from build123d import *

# Parameters (mm, degrees)
F1_DEPTH       = 600
F2_R           = 5
F3_R           = 5
F4_T1_DEPTH    = 611.3695297687
F5_SIZE        = 1
F7_D           = 2.5
F7_CBORE_D     = 6.5
F7_CBORE_DEPTH = 3


# Not quite as in the source:
# - a fillet or chamfer that OpenCascade refuses, or shapes differently, is made with other operations: its cross-section is extruded or revolved along the edge and cut away or added


with BuildPart() as f1:
    # F0 (on Front) → F1 (new body)
    with BuildSketch(Plane.XZ):
        Polygon((-100, 12.6136353192), (0, 12.6136353192), (0, 17.5048394176), (0, 17.6136353192), (-100, 17.6136353192), (-125.63551, 43.2491453192), (-130.63551, 48.2491453192), (-155.818130374, 48.7903356552), (-155.818130374, 43.2491453192), (-130.63551, 43.2491453192), align=None)
    extrude(amount=F1_DEPTH)

    # F2
    f2_edges = [f1.edges().sort_by_distance(p)[0] for p in [
        (-130.63551, -300, 48.249145),
        (-100, -300, 17.613635),
    ]]
    fillet(f2_edges, radius=F2_R)

    # F3
    f3_edges = [f1.edges().sort_by_distance(p)[0] for p in [
        (-130.63551, -300, 43.249145),
        (-100, -300, 12.613635),
        (-155.81813, -300, 43.249145),
    ]]
    fillet(f3_edges, radius=F3_R)

    # F4: fillet of radius 5 on 1 edges, made by hand

    # F4_s2 → F4_t1 (cut)
    with BuildSketch(Plane.XZ.offset(-5.6847648844)):
        with BuildLine():
            ThreePointArc((-155.818130374, 48.2491453192), (-154.7104681905, 48.6293523426), (-153.5447493368, 48.7414792682))
            Line((-153.5447493368, 48.7414792682), (-155.818130374, 48.7903356552))
            Line((-155.818130374, 48.7903356552), (-155.818130374, 48.2491453192))
        make_face()
    extrude(amount=F4_T1_DEPTH, mode=Mode.SUBTRACT)

    # F5
    f5_edges = [f1.edges().sort_by_distance(p)[0] for p in [
        (-48.964466, 0, 17.613635),
        (-48.964466, 0, 12.613635),
        (-115.317755, 0, 27.93139),
        (-130.793161, 0, 42.868543),
        (-141.762354, 0, 43.249145),
        (-154.353664, 0, 44.713611),
        (-143.094103, 0, 48.516888),
        (-130.787949, 0, 47.892026),
        (-154.710468, 0, 48.629352),
        (-99.842349, 0, 12.994238),
        (-99.842349, 0, 17.994238),
        (-115.339908, 0, 32.953543),
        (0, 0, 15.113635),
    ]]
    chamfer(f5_edges, length=F5_SIZE)

    # F7 (through all)
    with Locations(Plane.XY.offset(17.6136353192)):
        with Locations((-48.9644660941, -73), (-48.9644660941, -527)):
            CounterBoreHole(F7_D / 2, F7_CBORE_D / 2, F7_CBORE_DEPTH)


solid = f1.part
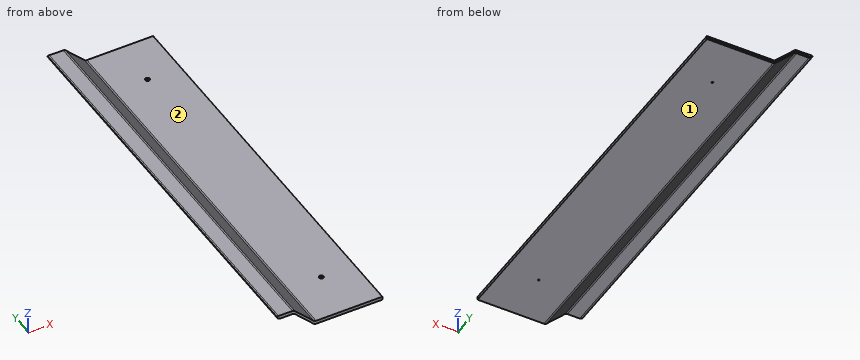
CAD build for the part. Positions are in the model's coordinates, mm. Face numbers are marked on the shaded views. A direction names the side the tool comes from. Round coordinates to 2 decimals unless told otherwise and drop trailing zeros. Loops run counter-clockwise (first coordinate to the right, second up) from the corner with the lowest first, then second, coordinate; pieces in that order, holes last.
(1) Cut at C-C (z = 24.5). Give the cut face in (x, y).
(2) Drop flat-ended pins along their axis: pin 1 (14.5 mm diameter, centred on x = -142.5, y = -297.5, fed in from -Z); pin 2 (1.5 mm diameter, centred on y = -432.5, z = 35, fed in from +X); pin 3 (3 mm diameter, centred on x = -48.96, y = -527, fed in from +Z); pin 4 (1.5 mm diameter, centred on x = -48.96, y = -73, fed in from -Z). Give the stop position or say it passes through.
(3) Cut at A-A (y = -363.5). Give the cut face in (x, z), plus the area to 3 significant figures.
(4) Which spindle directions (+Z, -Z, +X, -X, +Y, -Y) get a long thin tool onto all of the face, cutting with end or side? Do the marked faces 1 and 2. Say none if no direction does.
(5) Cut at B-B (x = -82.5). Give the cut face in (y, z), plus the area to 3 significant figures.
(6) Wall check: line 1 along Z through (x, y) = (-39, -316); line 2 along Z through (x, y) = (-99, -542); line 3 along X through (y, z) = (-129, 20). Give the ranges that are in metal, low to high.
Findings below:
1. outline: (-111.89, -600) - (-106.89, -600) - (-106.89, -1) - (-108.3, 0) - (-110.47, 0) - (-111.89, -1) - close
2. pin 1: stops at z = 43.25
2. pin 2: stops at x = -116.64
2. pin 3: stops at z = 14.61
2. pin 4: passes through
3. outline: (-155.82, 48.25) arc R5 ccw to (-150.82, 43.25) - (-132.71, 43.25) arc R5 cw to (-129.17, 41.78) - (-101.46, 14.08) arc R5 ccw to (-97.93, 12.61) - (0, 12.61) - (0, 17.61) - (-97.93, 17.61) arc R5 cw to (-101.46, 19.08) - (-129.22, 46.83) arc R5 ccw to (-132.64, 48.29) - (-153.54, 48.74) arc R5 ccw to start
3. area: 780 mm2
4. face 1: -Z, +X, -X, +Y, -Y
4. face 2: +Z, +X, +Y, -Y
5. outline: (-600, 12.61) - (-1, 12.61) - (0, 13.61) - (0, 16.61) - (-1, 17.61) - (-600, 17.61) - close
5. area: 3,000 mm2
6. line 1: z = 12.61 to 17.61
6. line 2: z = 12.73 to 17.73
6. line 3: x = -107.39 to -102.39
